from build123d import *

# Parameters (mm, degrees)
BOSS_EXTRU_1_DEPTH           = 20
ENL_V_MAT_EXTRU_1_DEPTH      = 29.705400189
ENL_V_MAT_EXTRU_1_DEPTH_BACK = 29.705400189
ESQUISSE2_R                  = 4
ENL_V_MAT_EXTRU_2_DEPTH      = 29.178005607
ENL_V_MAT_EXTRU_2_DEPTH_BACK = 29.178005607
ESQUISSE3_R                  = 1.5


with BuildPart() as part:
    # Esquisse1 → Boss.-Extru.1 (new body)
    with BuildSketch(Plane.XY):
        Polygon((0, 0), (13, 0), (13, 3), (3, 3), (3, 18), (0, 18), align=None)
    extrude(amount=BOSS_EXTRU_1_DEPTH)

    # Esquisse2 → Enl_v. mat.-Extru.1 (cut, two sides: drawn at the far end of the back side and taken through both)
    with BuildSketch(Plane(origin=(3, 0, 0), x_dir=(0, 0, -1), z_dir=(1, 0, 0)).offset(-ENL_V_MAT_EXTRU_1_DEPTH_BACK)):
        with Locations(Location((-10, 9.6, 0), (0, 0, 90))):
            Circle(ESQUISSE2_R)
    extrude(amount=ENL_V_MAT_EXTRU_1_DEPTH + ENL_V_MAT_EXTRU_1_DEPTH_BACK, mode=Mode.SUBTRACT)

    # Esquisse3 → Enl_v. mat.-Extru.2 (cut, two sides: drawn at the far end of the back side and taken through both)
    with BuildSketch(Plane(origin=(0, 3, 0), x_dir=(1, 0, 0), z_dir=(0, 1, 0)).offset(-ENL_V_MAT_EXTRU_2_DEPTH_BACK)):
        with Locations(Location((8, -5, 0), (0, 0, 180))):
            Circle(ESQUISSE3_R)
        with Locations(Location((8, -15, 0), (0, 0, 180))):
            Circle(ESQUISSE3_R)
    extrude(amount=ENL_V_MAT_EXTRU_2_DEPTH + ENL_V_MAT_EXTRU_2_DEPTH_BACK, mode=Mode.SUBTRACT)


solid = part.part
Here's how the part is built. I have some questions about the finished solid (model axes, mm). A direction names the side the tool comes from. Give positions to 0.01 mm unless a question says otherwise; leave off trailing zeros. Order: outer loops, then holes, each group sorted by start corner. A loop starts at its lowest first (then second) coordinate and runs counter-clockwise, first axis right, second up. Notation, with made-up numbers: M 85.5,72.5 L 136.5,72.5 A22 ccw 136.5,109.5 Z; hole C 25,46.25 d1. An arc over 180 degrees is marked long. Answer as a JSON object with one key per item and string values. Group by question number.
1) Suppose I cut it at D-D, the plane z = 5. Write out the boundary of the cut face in (x, y).
2) Suppose I cut it at B-B, the plane y = 9.6. Write out the boundary of the cut face in (x, z), plus the area to 3 significant figures.
3) I'm going to push flat-ended pins straight in: pin 1 Ø1.5 at (x, y) = (11, 4) entering from -Z (1 decimal); pin 2 Ø1.5 at (x, z) = (8, 10) entering from +Y. Where does each tip first touch, or does it pass through?
4) Suppose I cut it at C-C, the plane x = 8.75. Write out the boundary of the cut face in (y, z), plus the area to 3 significant figures.
5) On a 3-axis mill with a long thin cutter (end or side, diameter ignored), from which of +Z, -Z, +X, -X, +Y, -Y can I reach the whole of each face in a straight line? I mean faces 5 (the flat face through (13, 1, 10)), 6 (the flat face through (3, 14, 10)). Say none if no direction works.
6) Suppose I cut it at A-A, the plane z = 10. Write out the boundary of the cut face in (x, y), plus the area to 3 significant figures.
7) We'd pull the mould along Y, two halves only. Please class faces 1 (the flat face through (0, 5, 10)), 2 (the flat face through (8, 3, 10)), 3 (the cylindrical face through (1.479, 13.415, 11.201)), 4 (the flat face through (6, 0, 10)): pulls with the +Y half, pulls with the -Y half, needs draft (parallel to the pull), parting line crosses it, or undercut.
8) Please list where these lines run through material, in increasing order: L1, parallel to X at y = 1.4, z = 5; L2, parallel to Z at x = 0.65, y = 9.6; L3, parallel to Y at x = 0.7, z = 10. Write a range as [from, to].
Results found:
{
 "1": {"outline": "M 0,0 L 6.5,0 L 6.5,3 L 3,3 L 3,18 L 0,18 Z; M 9.5,0 L 13,0 L 13,3 L 9.5,3 Z"},
 "2": {"outline": "M 0,0 L 3,0 L 3,6 L 0,6 Z; M 0,14 L 3,14 L 3,20 L 0,20 Z", "area": "36.0 mm²"},
 "3": {"pin 1": "through", "pin 2": "y = 3"},
 "4": {"outline": "M 0,0 L 3,0 L 3,3.7 L 0,3.7 Z; M 0,6.3 L 3,6.3 L 3,13.7 L 0,13.7 Z; M 0,16.3 L 3,16.3 L 3,20 L 0,20 Z", "area": "44.4 mm²"},
 "5": {"face 5": "+Z, -Z, +X, +Y, -Y", "face 6": "+Z, -Z, +X, +Y"},
 "6": {"outline": "M 0,0 L 13,0 L 13,3 L 3,3 L 3,5.6 L 0,5.6 Z; M 0,13.6 L 3,13.6 L 3,18 L 0,18 Z", "area": "60.0 mm²"},
 "7": {"face 1": "needs draft", "face 2": "pulls with the +Y half", "face 3": "undercut", "face 4": "pulls with the -Y half"},
 "8": {"L1": "[0, 6.5], [9.5, 13]", "L2": "[0, 6], [14, 20]", "L3": "[0, 5.6], [13.6, 18]"}
}
